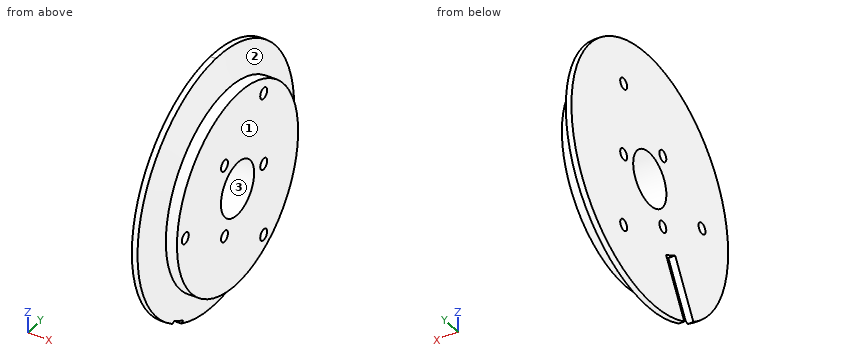
```python
from build123d import *

# Parameters (mm, degrees)
SKETCH5_R          = 7.94
CUT_EXTRUDE1_DEPTH = 54.633012222
SKETCH7_R          = 1.65
CUT_EXTRUDE3_DEPTH = 54.633012222
SKETCH6_W          = 2
SKETCH6_H          = 5
CUT_EXTRUDE2_DEPTH = 65.4


with BuildPart() as part:
    # Sketch3 → Revolve1 (revolve)
    with BuildSketch(Plane.XY, mode=Mode.PRIVATE) as revolve1_sk:
        Polygon((0, 0), (8, 0), (8, 29), (4.743746991, 29), (1.65, 37.5), (0, 37.5), align=None)
    revolve(revolve1_sk.sketch.rotate(Axis((0, 0, 0), (1, 0, 0)), 90), axis=Axis((0, 0, 0), (1, 0, 0)))

    # Sketch5 → Cut-Extrude1 (cut, through all)
    with BuildSketch(Plane(origin=(0, 0, 0), x_dir=(0, 0, -1), z_dir=(1, 0, 0))):
        Circle(SKETCH5_R)
    extrude(amount=CUT_EXTRUDE1_DEPTH, mode=Mode.SUBTRACT)

    # Sketch7 → Cut-Extrude3 (cut, through all)
    with BuildSketch(Plane(origin=(8, 0, 0), x_dir=(0, 0, -1), z_dir=(1, 0, 0))):
        with Locations((0, 12.5)):
            Circle(SKETCH7_R)
        with Locations((-10.825317547, -6.25)):
            Circle(SKETCH7_R)
        with Locations((10.825317547, -6.25)):
            Circle(SKETCH7_R)
        with Locations((-21.650635095, 12.5)):
            Circle(SKETCH7_R)
        with Locations((21.650635095, 12.5)):
            Circle(SKETCH7_R)
        with Locations((0, -25)):
            Circle(SKETCH7_R)
    extrude(amount=-CUT_EXTRUDE3_DEPTH, mode=Mode.SUBTRACT)

    # Sketch6 → Cut-Extrude2 (cut)
    with BuildSketch(Plane(origin=(0, -38.5, -0.866025404), x_dir=(1, 0, 0), z_dir=(0, -0.499999999999998, -0.8660254037844398))):
        with Locations((1, -32.908965344)):
            Rectangle(SKETCH6_W, SKETCH6_H)
    extrude(amount=CUT_EXTRUDE2_DEPTH, mode=Mode.SUBTRACT)


solid = part.part
```
CAD build for the part. Positions are in the model's coordinates, mm. Face numbers are marked on the shaded views. Give positions to 0.01 mm unless a question says otherwise; leave off trailing zeros. Loops run counter-clockwise (first coordinate to the right, second up) from the corner with the lowest first, then second, coordinate; pieces in that order, holes last. Notation, with made-up numbers: (-26.75, 85.25) - (15.25, 85.25) arc R18 ccw to (15.25, 107.25) - close; hole circle Ø3 at (-2.5, 17). An arc over 180 degrees is marked (long way). Put each result on its own line as item: value.
Q1. Probe line 1 along Y through (x, z) = (1.5, 0); line 2 along Z through (x, y) = (5.5, 12); line 3 along X through (y, z) = (-15.5, -22). List the from-to ranges inside material, lowest first.
Filled in:
line 1: y = -37.5 to -26.65, -23.35 to -7.94, 7.94 to 10.85, 14.15 to 37.5
line 2: z = -26.4 to -23.22, -20.08 to -1.57, 1.57 to 20.08, 23.22 to 26.4
line 3: x = 2 to 8
Q2. Mould opens along Z. For the marked faces 1, 2 and 3 say: pulls with the +Z half, pulls with the -Z half, needs draft (parallel to the pull), parting line crosses it, or undercut.
Filled in:
face 1: needs draft
face 2: parting line crosses it
face 3: undercut
Q3. Flat gauge pins, fed straight in: pin 1 (2.5 mm diameter, centred on y = 12.5, z = -21.65, fed in from -X); pin 2 (4 mm diameter, centred on x = 6.5, y = 28.5, fed in from +Z); pin 3 (4 mm diameter, centred on x = 1.5, z = 22, fed in from +Y); pin 4 (1.5 mm diameter, centred on x = 6.5, y = 24, fed in from +Z). Where does each tip first touch, or does it go through?
Filled in:
pin 1: passes through
pin 2: stops at z = 11.78
pin 3: stops at y = 31.72
pin 4: stops at z = 17.33
Q4. Slice it at B-B (x = 6). Give the cut face in (y, z), plus the area to 3 significant figures.
Filled in:
outline: circle Ø58 at (0, 0); hole circle Ø3.3 at (-25, 0); hole circle Ø15.88 at (0, 0); hole circle Ø3.3 at (-6.25, -10.83); hole circle Ø3.3 at (-6.25, 10.83); hole circle Ø3.3 at (12.5, -21.65); hole circle Ø3.3 at (12.5, 0); hole circle Ø3.3 at (12.5, 21.65)
area: 2,390 mm²
Q5. Slice it at A-A (z = 0). Give the cut face in (x, y), plus the area to 3 significant figures.
Filled in:
outline: (0, -37.5) - (1.65, -37.5) - (4.74, -29) - (8, -29) - (8, -26.65) - (0, -26.65) - close; (0, -23.35) - (8, -23.35) - (8, -7.94) - (0, -7.94) - close; (0, 7.94) - (8, 7.94) - (8, 10.85) - (0, 10.85) - close; (0, 14.15) - (8, 14.15) - (8, 29) - (4.74, 29) - (1.65, 37.5) - (0, 37.5) - close
area: 339 mm²
Q6. Slice it at C-C (y = 12.5). Give the number of separate pieces and of enclosed holes in the cut face, plus the area to 3 significant figures.
Filled in:
separate pieces: 4
enclosed holes: 0
area: 398 mm²
